Answer from the drawing. Dimensions are ordinates in mm from the lowest x, y and z of the part. A direction names the side the tool comes from. Coordinates: 2 decimals unless noted, no trailing zeros. Order: outer loops, then holes, each group sorted by start corner. A loop starts at its lowest first (then second) coordinate and runs counter-clockwise, first axis right, second up. Notation, with made-up numbers: (45, -13) -> (82, -13) arc R21 ccw to (82, 9) -> close; hole circle Ø3 at (19, -4). An arc over 180 degrees is marked (long way). Answer in a Markdown table with one row per item.
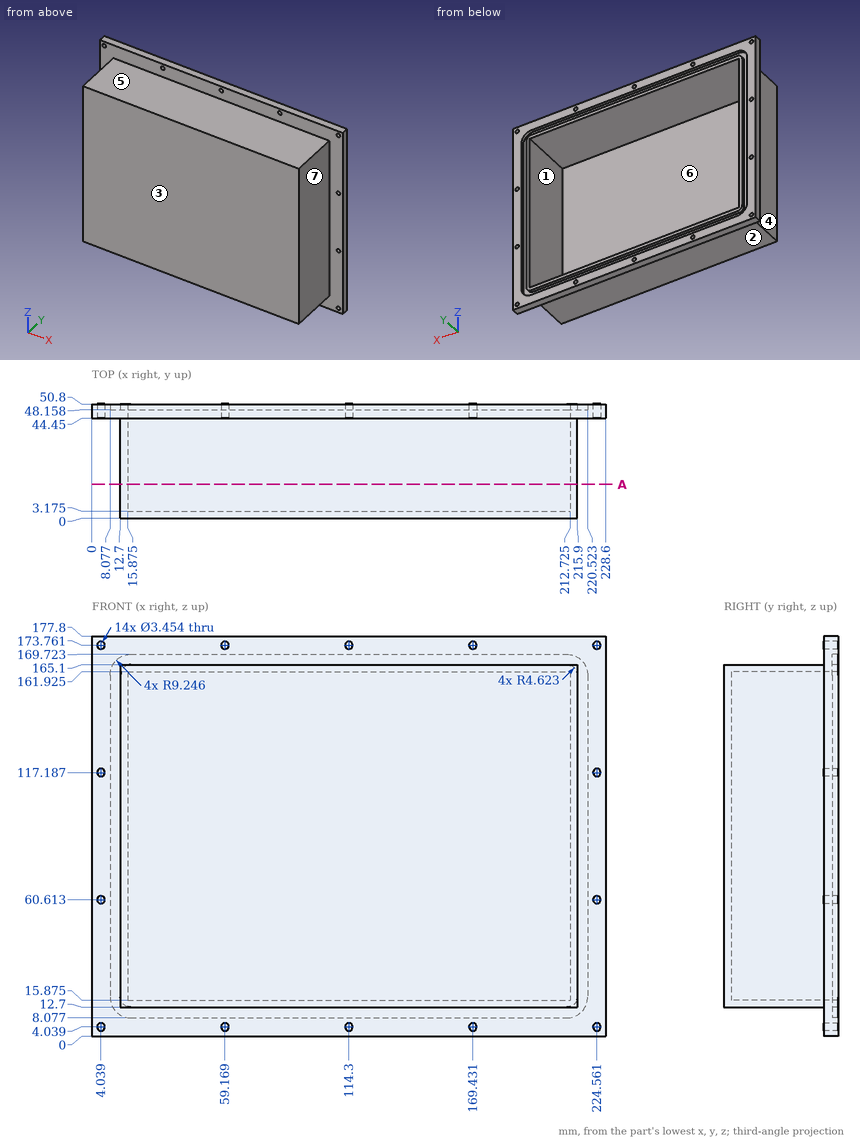
Q1. For the marked faces 1, 2, 3 and 4, determine the directions among +Z, -Z, +X, -X, +Y, -Y from which every point of the face is accessible in a straight line to the end or side of a thin tool.
Outcome:
| item | result |
|---|---|
| face 1 | +Y |
| face 2 | -Z, +X, -X, -Y |
| face 3 | +Z, -Z, +X, -X, -Y |
| face 4 | +Z, -Z, -X, -Y |
Q2. For a pull along Z with two mould halves and no side action, classify the marked faces 5, 6 and 7 as pulls with the +Z half, pulls with the -Z half, needs draft (parallel to the pull), parting line crosses it, or undercut.
Outcome:
| item | result |
|---|---|
| face 5 | pulls with the +Z half |
| face 6 | undercut |
| face 7 | needs draft |
Q3. Given pin 1 (4 mm diameter, centred on y = 7, z = 155, fed in from +X); pin 2 (12 mm diameter, centred on x = 157, z = 153, fed in from +Y) (3 decimals); pin 3 (12 mm diameter, centred on x = 62.5, z = 135.5, fed in from -Y); pin 4 (4.5 mm diameter, centred on x = 4.04, z = 60.61, fed in from -Y), each flat-ended and moving along its own axis, determine where each tip first touches the part or whether it passes through.
Outcome:
| item | result |
|---|---|
| pin 1 | x = 215.9 |
| pin 2 | y = 3.175 |
| pin 3 | y = 0 |
| pin 4 | y = 44.45 |
Q4. The part is cut by section A-A (y = 15). Write down the section's boundary in (x, z) (1 decimal), then the cut area to 3 significant figures.
Outcome:
| item | result |
|---|---|
| outline | (12.7, 12.7) -> (215.9, 12.7) -> (215.9, 165.1) -> (12.7, 165.1) -> close; hole (15.9, 15.9) -> (212.7, 15.9) -> (212.7, 161.9) -> (15.9, 161.9) -> close |
| area | 2,220 mm² |
Q5. Consider line 1 (Z direction, x = 194.5, y = 15.5) (1 decimal); line 2 (X direction, y = 48, z = 28) (1 decimal); line 3 (X direction, y = 8, z = 33) (1 decimal). Determine where each line is inside the solid, lowest interval first.
Outcome:
| item | result |
|---|---|
| line 1 | 12.7 to 15.9, 161.9 to 165.1 |
| line 2 | 0 to 15.9, 212.7 to 228.6 |
| line 3 | 12.7 to 15.9, 212.7 to 215.9 |
